Build history of the part. All positions in model axes, mm. A direction names the side the tool comes from. Round coordinates to 2 decimals unless told otherwise and drop trailing zeros. Write each loop counter-clockwise with the first axis right and the second up, starting at its lowest first coordinate (ties: lowest second). Pieces come first, ordered by that corner, then holes. Notation, with made-up numbers: (22, 49) -> (43, 49) arc R17 cw to (43, 63) -> close; hole circle Ø4 at (-22, 89.5). An arc over 180 degrees is marked (long way). Return JSON: item names as keys, results as strings.
Autodesk Inventor part; units mm, degrees
ref_plane "YZ Plane" through (0, 0, 0) normal (1, 0, 0) x (0, 1, 0)
ref_plane "XZ Plane" through (0, 0, 0) normal (0, 1, 0) x (-1, 0, 0)
ref_plane "XY Plane" through (0, 0, 0) normal (0, 0, 1) x (1, 0, 0)
sketch "Sketch1" plane through (0, 0, 0) normal (0, 0, 1) x (1, 0, 0)
  arc A0 (-25.4018, -15) -> (25.4018, -15) centre (0, 0) ccw
  line L0 (2.5, -32) -> (2.5, -39)
  line L1 (2.5, -39) -> (-2.5, -39)
  line L2 (-2.5, -39) -> (-2.5, -32)
  line L3 (-2.5, -32) -> (-2.5, -31.9022)
  line L4 (2.5, -32) -> (2.5, -31.9022)
  arc A1 (-28.2666, -15) -> (-2.5, -31.9022) centre (0, 0) ccw
  arc A2 (2.5, -31.9022) -> (28.2666, -15) centre (0, 0) ccw
  arc A3 (-27.7534, -10) -> (27.7534, -10) centre (0, 0) ccw
  line L5 (-27.7534, -10) -> (-30.3974, -10)
  line L6 (27.7534, -10) -> (30.3974, -10)
  arc A4 (-30.3974, -10) -> (-2.5, -31.9022) centre (0, 0) ccw
  arc A5 (2.5, -31.9022) -> (30.3974, -10) centre (0, 0) ccw
  point P0 (25.4018, -15)
  point P1 (-28.2666, -15)
  dimension "d43" = 5
  dimension "d64" = 7
extrude "Extrusion6" add sketch "Sketch1" along normal blind 5
properties part number "Clip_TestFitV1"
Q1. Saw through at B-B on z = 3.9. List the corners of the cut face in (x, y), then the cut area to 3 significant figures.
Verdict:
{"outline": "(-30.4, -10) arc R32 ccw to (-28.27, -15) arc R32 ccw to (-2.5, -31.9) -> (-2.5, -39) -> (2.5, -39) -> (2.5, -31.9) arc R32 ccw to (28.27, -15) arc R32 ccw to (30.4, -10) -> (27.75, -10) arc R29.5 cw to (-27.75, -10) -> close", "area": "226 mm²"}
Q2. Saw through at D-D on x = 19.5. List the corners of the cut face in (y, z), then the cut area to 3 significant figures.
Verdict:
{"outline": "(-25.37, 0) -> (-22.14, 0) -> (-22.14, 5) -> (-25.37, 5) -> close", "area": "16.2 mm²"}
Q3. Pin check, flat tips, straight feed: pin 1 Ø1 at (y, z) = (-15, 3) entering from -X; pin 2 Ø3 at (x, z) = (9, 2.5) entering from -Y; pin 3 Ø2.5 at (y, z) = (-36.5, 2) entering from +X. Stop position of each tip, or through.
Verdict:
{"pin 1": "stops at x = -28.53", "pin 2": "stops at y = -31.11", "pin 3": "stops at x = 2.5"}
Q4. 3-axis set-ups, long thin cutter, end or side, ignore diameter. For faces 4 (the flat face through (0, -30, 0)), 5 (the flat face through (-2.5, -36, 2)), 6 (the flat face through (2.5, -35, 2)): which of +Z, -Z, +X, -X, +Y, -Y reach the whole face in a straight line?
Verdict:
{"face 4": "-Z, +X, -X, +Y, -Y", "face 5": "+Z, -Z, -X, -Y", "face 6": "+Z, -Z, +X, -Y"}
Q5. Saw through at C-C on y = -22.75. List the corners of the cut face in (x, z).
Verdict:
{"outline": "(-22.5, 0) -> (-18.78, 0) -> (-18.78, 5) -> (-22.5, 5) -> close; (18.78, 0) -> (22.5, 0) -> (22.5, 5) -> (18.78, 5) -> close"}
Q6. Wall check: L1, parallel to X at y = -36.25, z = 4; L2, parallel to X at y = -17.5, z = 2.7; L3, parallel to Y at x = 15, z = 1.8. Give the ranges that are in metal, low to high.
Verdict:
{"L1": "x = -2.5 to 2.5", "L2": "x = -26.79 to -23.75, 23.75 to 26.79", "L3": "y = -28.27 to -25.4"}
Q7. Two-plate mould, pull along X, no slides. Class faces 1 (the flat face through (0, -30, 5)), 2 (the cylindrical face through (-17.36, -26.88, 2.46)), 3 (the cylindrical face through (17.74, -26.633, 2.465)): +X half, -X half, draft (parallel to the pull), parting line (faces both ways), or undercut.
Verdict:
{"face 1": "draft", "face 2": "-X half", "face 3": "+X half"}
Q8. Saw through at A-A on y = -25.75. List the corners of the cut face in (x, z).
Verdict:
{"outline": "(-19, 0) -> (-14.39, 0) -> (-14.39, 5) -> (-19, 5) -> close; (14.39, 0) -> (19, 0) -> (19, 5) -> (14.39, 5) -> close"}
